The listing builds one solid part. Answer for the finished solid, in the listing's coordinates (mm). Give positions to 0.01 mm unless a question says otherwise; leave off trailing zeros. Order: outer loops, then holes, each group sorted by start corner. A loop starts at its lowest first (then second) coordinate and runs counter-clockwise, first axis right, second up. Notation, with made-up numbers: (70, 12.5) - (88, 12.5) arc R24 ccw to (88, 26.5) - close; hole circle Ø5 at (40.25, 14.5). An arc over 180 degrees is marked (long way). Answer as CSV lines item,"result". Start each with the question number.
1. Section C-C on z = 20.5 is taken. Give the vertices of the cut face in (x, y).
2. Consider line 1 along Y through (x, z) = (2.2, 30.75); line 2 along Y through (x, z) = (1.6, 32); line 3 along Y through (x, z) = (1.2, 21.5). Determine where each line is inside the solid, lowest interval first. Write a range as [from, to].
3. Determine the mould class of faces 1 (the cylindrical face through (1.48, -88.4, 30.75)), 2 (the flat face through (3, -9, 31)), 3 (the flat face through (1, -9, 18.119)) for opening direction Z: +Z half, -Z half, draft (parallel to the pull), parting line (faces both ways), or undercut.
4. Section A-A on x = 1.7 is taken. Give the vertices of the cut face in (y, z), and give its area (3 significant figures).
5. Section B-B on z = 39.5 is taken. Give the vertices of the cut face in (x, y).
6. A flat-ended cylindrical pin translates along its axis: pin 1 (5 mm diameter, centred on y = -85.4, z = 30.62, fed in from -X) (3 decimals). Find the tip coordinate at first contact, or state that the pin passes through.
from build123d import *

# Parameters (mm, degrees)
F0_R     = 3
F1_DEPTH = 3


with BuildPart() as f1:
    # F0 (on Right) → F1 (new body)
    with BuildSketch(Plane.YZ):
        with BuildLine():
            Line((69.598682, 43.118995), (-85.401318, 43.118995))
            ThreePointArc((-85.401318, 43.118995), (-94.240152, 39.45783), (-97.901318, 30.618995))
            ThreePointArc((-97.901318, 30.618995), (-94.240152, 21.78016), (-85.401318, 18.118995))
            Line((-85.401318, 18.118995), (69.598682, 18.118995))
            ThreePointArc((69.598682, 18.118995), (78.437517, 21.78016), (82.098682, 30.618995))
            ThreePointArc((82.098682, 30.618995), (78.437517, 39.45783), (69.598682, 43.118995))
        make_face()
        with Locations((-85.401318, 30.618995)):
            Circle(F0_R, mode=Mode.SUBTRACT)
        with Locations((69.598682, 30.618995)):
            Circle(F0_R, mode=Mode.SUBTRACT)
    extrude(amount=F1_DEPTH)


solid = f1.part
Checks:
1,outline,"(0, -92.74) - (3, -92.74) - (3, 76.94) - (0, 76.94) - close"
2,line 1,"y = [-97.9, -88.4], [-82.4, 66.6], [72.6, 82.1]"
2,line 2,"y = [-97.82, -88.06], [-82.74, 66.94], [72.26, 82.02]"
2,line 3,"y = [-93.95, 78.15]"
3,face 1,"undercut"
3,face 2,"draft"
3,face 3,"-Z half"
4,outline,"(-97.9, 30.62) arc R12.5 ccw to (-85.4, 18.12) - (69.6, 18.12) arc R12.5 ccw to (82.1, 30.62) arc R12.5 ccw to (69.6, 43.12) - (-85.4, 43.12) arc R12.5 ccw to start; hole circle Ø6 at (-85.4, 30.62); hole circle Ø6 at (69.6, 30.62)"
4,area,"4,310 mm²"
5,outline,"(0, -94.2) - (3, -94.2) - (3, 78.4) - (0, 78.4) - close"
6,pin 1,"passes through"
